Can you work these out from the drawing? Everything is in mm from the part's minimum corner. A direction names the side the tool comes from. Coordinates: 2 decimals unless noted, no trailing zeros. Write each loop counter-clockwise with the first axis right and the second up, starting at its lowest first coordinate (ties: lowest second). Pieces come first, ordered by that corner, then holes. Notation, with made-up numbers: (60, -31) -> (107, -31) arc R12 ccw to (107, -22) -> close; hole circle Ø3 at (-11, -37). An arc over 180 degrees is marked (long way). Use a Markdown table: item, result. Add a question column.
Item 1: If I drill on line 1 along Z through (x, y) = (91, 32); line 2 along Y through (x, z) = (20.5, 47), over which ranges is the centre line in solid material (lowest first)? Write a range as from..to.
Item 2: Imagine slicing it at B-B, the plane x = 248.5. Write out the boundary of the cut face in (y, z).
Item 3: Will these pins go through, and if not, where does the flat tip stop? pin 1 Ø12 at (x, y) = (133.5, 33.5) entering from -Z; pin 2 Ø8 at (x, z) = (172.5, 73.5) entering from +Y.
Item 4: Imagine slicing it at A-A, the plane y = 27. Write out the boundary of the cut face in (x, z).
Item 5: On a 3-axis mill with a long thin cutter (end or side, diameter ignored), from which of +Z, -Z, +X, -X, +Y, -Y can I reach the whole of each face in a straight line? I mean the marked faces 4 and 5. Say none if no direction works.
Item 6: If we mould it in two halves opening along Z, with no side actions, what happens to the marked faces 1, 2 and 3? For each: pulls with the +Z half, pulls with the -Z half, needs draft (parallel to the pull), parting line crosses it, or undercut.
Item 7: Imagine slicing it at C-C, the plane z = 88. Write out the boundary of the cut face in (x, y).
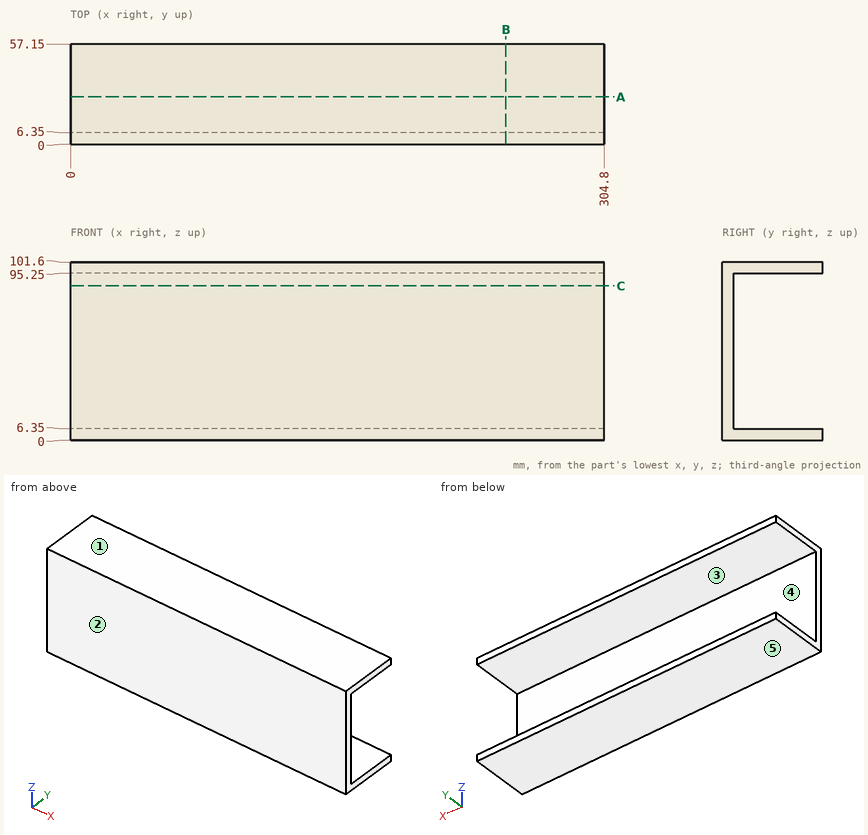
Ans:
| question | item | result |
|---|---|---|
| 1 | line 1 | z = 0..6.35, 95.25..101.6 |
| 1 | line 2 | y = 0..6.35 |
| 2 | outline | (0, 0) -> (57.15, 0) -> (57.15, 6.35) -> (6.35, 6.35) -> (6.35, 95.25) -> (57.15, 95.25) -> (57.15, 101.6) -> (0, 101.6) -> close |
| 3 | pin 1 | stops at z = 0 |
| 3 | pin 2 | stops at y = 6.35 |
| 4 | outline | (0, 0) -> (304.8, 0) -> (304.8, 6.35) -> (0, 6.35) -> close; (0, 95.25) -> (304.8, 95.25) -> (304.8, 101.6) -> (0, 101.6) -> close |
| 5 | face 4 | +X, -X, +Y |
| 5 | face 5 | -Z, +X, -X, +Y, -Y |
| 6 | face 1 | pulls with the +Z half |
| 6 | face 2 | needs draft |
| 6 | face 3 | undercut |
| 7 | outline | (0, 0) -> (304.8, 0) -> (304.8, 6.35) -> (0, 6.35) -> close |
